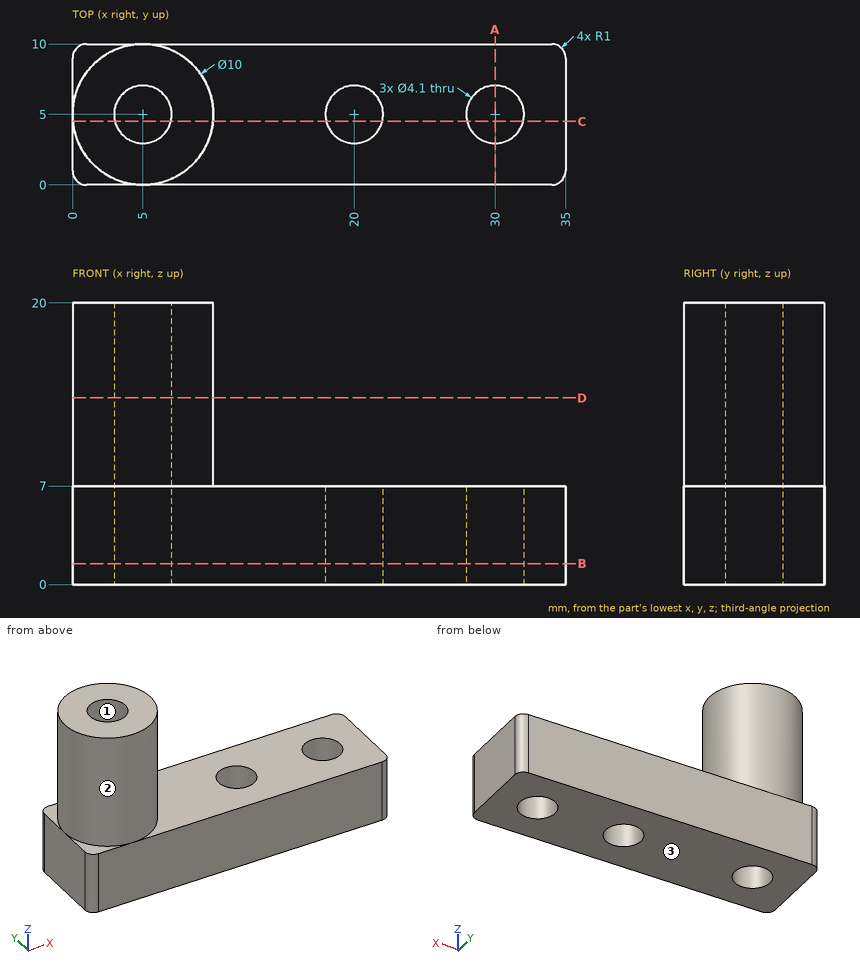
Could you check a few things on this drawing? It's one solid part, dimensions in mm from its lowest x, y, z. Give positions to 0.01 mm unless a question says otherwise; leave off trailing zeros. Write each loop counter-clockwise with the first axis right and the second up, starting at its lowest first coordinate (ties: lowest second). Pieces come first, ordered by that corner, then holes. Notation, with made-up numbers: (11, -26) -> (44, -26) arc R26 ccw to (44, -7) -> close; hole circle Ø2 at (15.5, 31). An arc over 180 degrees is marked (long way). Answer as CSV lines item,"result". Start each with the question number.
(1) I'm going to push flat-ended pins straight in: pin 1 Ø4 at (y, z) = (1.5, 14.5) entering from +X; pin 2 Ø2 at (x, y) = (13, 2) entering from +Z. Where does each tip first touch, or does it pass through?
(2) If we section it at D-D, the plane z = 13.25: Write out the boundary of the cut face in (x, y).
(3) If we section it at C-C, the plane y = 4.5: Give the number of separate pieces and of enclosed holes in the cut face, and give its area (3 significant figures).
(4) If we mould it in two halves opening along Y, with no side actions, what happens to the marked faces 1, 2 and 3? For each: +Y half, -Y half, draft (parallel to the pull), parting line (faces both ways), or undercut.
(5) If we section it at A-A, the plane x = 30: Write out the boundary of the cut face in (y, z).
(6) Please list where these lines run through material, in increasing order: line 1 (Y direction, x = 20, z = 1.5); line 2 (Z direction, x = 32.5, y = 7.5); line 3 (X direction, y = 4, z = 18.25).
(7) If we section it at B-B, the plane z = 1.5: Write out the boundary of the cut face in (x, y), and give its area (3 significant figures).
Answer list:
1,pin 1,"x = 9.77"
1,pin 2,"z = 7"
2,outline,"circle Ø10 at (5, 5); hole circle Ø4.1 at (5, 5)"
3,separate pieces,"4"
3,enclosed holes,"0"
3,area,"239 mm^2"
4,face 1,"undercut"
4,face 2,"parting line"
4,face 3,"draft"
5,outline,"(0, 0) -> (2.95, 0) -> (2.95, 7) -> (0, 7) -> close; (7.05, 0) -> (10, 0) -> (10, 7) -> (7.05, 7) -> close"
6,line 1,"0 to 2.95, 7.05 to 10"
6,line 2,"0 to 7"
6,line 3,"0.1 to 3.21, 6.79 to 9.9"
7,outline,"(0, 1) arc R1 ccw to (1, 0) -> (34, 0) arc R1 ccw to (35, 1) -> (35, 9) arc R1 ccw to (34, 10) -> (1, 10) arc R1 ccw to (0, 9) -> close; hole circle Ø4.1 at (5, 5); hole circle Ø4.1 at (20, 5); hole circle Ø4.1 at (30, 5)"
7,area,"310 mm^2"
